```python
from build123d import *

# Parameters (mm, degrees)
SKETCH_2_W             = 20
SKETCH_2_H             = 10
EXTRUDE_1_DEPTH        = 55.75
SKETCH_3_W             = 20
SKETCH_3_H             = 10
SKETCH_3_R             = 2.75
SKETCH_3_W_2           = 10
EXTRUDE_2_DEPTH        = 4
FILLET_1_R             = 3
FILLET_1_OF_MIRROR_1_R = 3
FILLET_2_R             = 3


with BuildPart() as part:
    # 草图2 → 凸台-拉伸1 (new, symmetric)
    with BuildSketch(Plane(origin=(0, 0, 0), x_dir=(0, 0, -1), z_dir=(1, 0, 0))):
        Rectangle(SKETCH_2_W, SKETCH_2_H)
    extrude(amount=EXTRUDE_1_DEPTH, both=True)

    # 草图3 → 凸台-拉伸2 (add)
    # profile 1 of 3: a face of its own
    with BuildSketch(Plane(origin=(49.75, 0, 0), x_dir=(0, 0, -1), z_dir=(1, 0, 0))):
        with Locations((0, 10)):
            Rectangle(SKETCH_3_W, SKETCH_3_H)
        with Locations((0, 10)):
            Circle(SKETCH_3_R, mode=Mode.SUBTRACT)
    # profile 2 of 3: a face of its own
    with BuildSketch(Plane(origin=(49.75, 0, 0), x_dir=(0, 0, -1), z_dir=(1, 0, 0))):
        with Locations((15, 0)):
            Rectangle(SKETCH_3_W_2, SKETCH_3_H)
        with Locations((15, 0)):
            Circle(SKETCH_3_R, mode=Mode.SUBTRACT)
    # profile 3 of 3: a face of its own
    with BuildSketch(Plane(origin=(49.75, 0, 0), x_dir=(0, 0, -1), z_dir=(1, 0, 0))):
        with Locations((-15, 0)):
            Rectangle(SKETCH_3_W_2, SKETCH_3_H)
        with Locations((-15, 0)):
            Circle(SKETCH_3_R, mode=Mode.SUBTRACT)
    extrude_2 = extrude(amount=-EXTRUDE_2_DEPTH)

    # 圆角1
    fillet_1_edges = [part.edges().sort_by_distance(p)[0] for p in [
        (47.75, 15, 10),
        (47.75, 15, -10),
        (47.75, 5, -20),
        (47.75, 5, 20),
    ]]
    fillet(fillet_1_edges, radius=FILLET_1_R)

    # 镜向1: 凸台-拉伸2 across plane
    add(extrude_2.mirror(Plane(origin=(0, 0, 0), x_dir=(0, 0, 1), z_dir=(1, 0, 0))))

    # 圆角1 of 镜向1
    fillet_1_of_mirror_1_edges = [part.edges().sort_by_distance(p)[0] for p in [
        (-47.75, 15, 10),
        (-47.75, 15, -10),
        (-47.75, 5, -20),
        (-47.75, 5, 20),
    ]]
    fillet(fillet_1_of_mirror_1_edges, radius=FILLET_1_OF_MIRROR_1_R)

    # 圆角2
    # the kernel refuses this fillet: 3 mm, written as the material it takes off along each edge
    with BuildSketch(Plane(origin=(63.25, 5, 10), x_dir=(0, -1, 0), z_dir=(-1, 0, 0)), Plane(origin=(49.75, 5, -10), x_dir=(0, -1, 0), z_dir=(1, 0, 0)), Plane(origin=(-49.75, 5, 10), x_dir=(0, -1, 0), z_dir=(-1, 0, 0)), Plane(origin=(-63.25, 5, -10), x_dir=(0, -1, 0), z_dir=(1, 0, 0))) as fillet_2_piece_1:
        with BuildLine():
            CenterArc((FILLET_2_R, -FILLET_2_R), FILLET_2_R, 90, 90)
            Line((0, -FILLET_2_R), (0, 0))
            Line((0, 0), (FILLET_2_R, 0))
        make_face()
    extrude(amount=13.5, mode=Mode.SUBTRACT)


solid = part.part
```
Check sheet for the modelled part. Datum: model origin and axes. Units: mm. A direction names the side the tool comes from. Round coordinates to 2 decimals unless told otherwise and drop trailing zeros. Order: outer loops, then holes, each group sorted by start corner. A loop starts at its lowest first (then second) coordinate and runs counter-clockwise, first axis right, second up. Notation, with made-up numbers: (79.25, 72.5) -> (90.25, 72.5) arc R12 ccw to (90.25, 78.5) -> close; hole circle Ø7 at (52.25, -2.5). An arc over 180 degrees is marked (long way). One line per item, written item: value. Start each with the question number.
Q1. Mould release check, pull along X, two halves, no side actions. Record for faces 6 (the face through (-55.75, 0, 0)), 7 (the face through (45.75, -2.2, 12.8)), 8 (the face through (-45.75, 7.8, 2.4)), 9 (the face through (47.72, 14.14, -9.1)): pulls with the +X half, pulls with the -X half, needs draft (parallel to the pull), parting line crosses it, or undercut.
Q2. Gauge pin test, flat ends, axial feed: pin 1 Ø3 at (x, y) = (53, -3) entering from +Z; pin 2 Ø1.8 at (x, z) = (-54, 3) entering from +Y; pin 3 Ø9 at (y, z) = (0, 15) entering from +X. Record the tip position at first contact, or that the pin passes through.
Q3. Set-up check for faces 1 (the face through (-53, -2, -10)), 2 (the face through (48, 8, 10)), 3 (the face through (53, 5, 0)), 4 (the face through (1, 5, 0)), 5 (the face through (48, 8, -10)): record each of +Z, -Z, +X, -X, +Y, -Y from which the full face is reachable in a straight line by a thin tool's end or side.
Q4. Cross-section at D-D (y = 0). Give the number of separate pieces and of enclosed holes in the cut face, and give its area (3 significant figures).
Q5. Thickness scan on line 1 (Y direction, x = -47.15, z = 0); line 2 (X direction, y = 8, z = -9); line 3 (Y direction, x = -48, z = -15). Record the ranges inside material, lowest first.
Q6. Cross-section at B-B (y = 10). Record the boundary of the cut face in (x, z).
Q7. Cross-section at C-C (z = 0). Record the boundary of the cut face in (x, y), and give its area (3 significant figures).
Q8. Cross-section at A-A (z = 15). Record the boundary of the cut face in (x, y), and give its area (3 significant figures).
Completed:
1. face 6: pulls with the -X half
1. face 7: undercut
1. face 8: undercut
1. face 9: needs draft
2. pin 1: stops at z = 10
2. pin 2: stops at y = 5
2. pin 3: stops at x = 49.75
3. face 1: -Z, -X, +Y, -Y
3. face 2: +Z, +X, -X, +Y
3. face 3: +Z, -Z, +X, +Y
3. face 4: +Z, -Z, +Y
3. face 5: -Z, +X, -X, +Y
4. separate pieces: 5
4. enclosed holes: 0
4. area: 2,300 mm²
5. line 1: y = -5 to 7.25, 12.75 to 15
5. line 2: x = -49.75 to -45.75, 45.75 to 49.75
5. line 3: y = -5 to -2.75, 2.75 to 5
6. outline: (-49.75, -10) -> (-45.75, -10) -> (-45.75, -2.75) -> (-49.75, -2.75) -> close; (-49.75, 2.75) -> (-45.75, 2.75) -> (-45.75, 10) -> (-49.75, 10) -> close; (45.75, -10) -> (49.75, -10) -> (49.75, -2.75) -> (45.75, -2.75) -> close; (45.75, 2.75) -> (49.75, 2.75) -> (49.75, 10) -> (45.75, 10) -> close
7. outline: (-55.75, -5) -> (55.75, -5) -> (55.75, 5) -> (49.75, 5) -> (49.75, 7.25) -> (45.75, 7.25) -> (45.75, 5) -> (-45.75, 5) -> (-45.75, 7.25) -> (-49.75, 7.25) -> (-49.75, 5) -> (-55.75, 5) -> close; (-49.75, 12.75) -> (-45.75, 12.75) -> (-45.75, 15) -> (-49.75, 15) -> close; (45.75, 12.75) -> (49.75, 12.75) -> (49.75, 15) -> (45.75, 15) -> close
7. area: 1,150 mm²
8. outline: (-49.75, -5) -> (-45.75, -5) -> (-45.75, -2.75) -> (-49.75, -2.75) -> close; (-49.75, 2.75) -> (-45.75, 2.75) -> (-45.75, 5) -> (-49.75, 5) -> close; (45.75, -5) -> (49.75, -5) -> (49.75, -2.75) -> (45.75, -2.75) -> close; (45.75, 2.75) -> (49.75, 2.75) -> (49.75, 5) -> (45.75, 5) -> close
8. area: 36.0 mm²
